For this review, take the finished solid that the model builds, in its own axes (mm). A direction names the side the tool comes from. Coordinates: 2 decimals unless noted, no trailing zeros. Order: outer loops, then holes, each group sorted by start corner. A loop starts at its lowest first (then second) coordinate and runs counter-clockwise, first axis right, second up. Notation, with made-up numbers: (35.25, 55) -> (46.25, 55) arc R11 ccw to (46.25, 66) -> close; hole circle Ø10 at (29, 6.5). An arc over 180 degrees is marked (long way). Answer as a JSON object with one key per item and string values. Group by question number.
1) Add section C-C, the plane z = -45.5. Write out the cut boundary in (x, y), then the cut area to 3 significant figures.
2) Machinability: for faces 1 (the flat face through (12, 22, -23)), 2 (the flat face through (0, 10, -62)), 3 (the flat face through (6, 20, -96)), which of the approach directions +Z, -Z, +X, -X, +Y, -Y give a long, thin tool a straight path to every point of the face, cutting with its end or side? Answer none if there is none.
3) Add section A-A, the plane y = 17. Write out the cut boundary in (x, z).
4) Draft analysis for pull direction Z (two halves, no side actions). For faces 4 (the flat face through (125, 13, -126)), 5 (the flat face through (125, 27, -5)), 6 (the flat face through (6, 20, -30)), state which applies: +Z half, -Z half, draft (parallel to the pull), parting line (faces both ways), or undercut.
5) Wall thickness on L1, parallel to X at y = 23.25, z = -28.5; L2, parallel to Z at x = 67, y = 25.5; L3, parallel to Z at x = 108.5, y = 17.5: over which ranges is each line inside the solid? List them lowest first.
6) For pin 1 (7 mm diameter, centred on x = 155, z = -17.5, fed in from +Y); pin 2 (12 mm diameter, centred on x = 116, z = -75, fed in from +Y), all flat-tipped, find the tip position at first contact; note any pin that passes through.
7) Add section B-B, the plane x = 154.5. Write out the cut boundary in (y, z).
from build123d import *

# Parameters (mm, degrees)
SKETCH1_W           = 253
SKETCH1_H           = 126
BOSS_EXTRUDE1_DEPTH = 27
SKETCH2_W           = 229
SKETCH2_H           = 102
CUT_EXTRUDE1_DEPTH  = 7
SKETCH3_W           = 229
SKETCH3_H           = 85
CUT_EXTRUDE2_DEPTH  = 7
SKETCH4_W           = 12
SKETCH4_H           = 66
CUT_EXTRUDE3_DEPTH  = 14
SKETCH5_W           = 12
SKETCH5_H           = 66
CUT_EXTRUDE4_DEPTH  = 14
CUT_EXTRUDE5_DEPTH  = 7
FILLET1_R           = 2.5


with BuildPart() as part:
    # Sketch1 → Boss-Extrude1 (new body)
    with BuildSketch(Plane(origin=(0, 0, 0), x_dir=(1, 0, 0), z_dir=(0, 1, 0))):
        with Locations((126.5, 63)):
            Rectangle(SKETCH1_W, SKETCH1_H)
    extrude(amount=BOSS_EXTRUDE1_DEPTH)

    # Sketch2 → Cut-Extrude1 (cut)
    with BuildSketch(Plane(origin=(0, 27, 0), x_dir=(1, 0, 0), z_dir=(0, 1, 0))):
        with Locations((126.5, 63)):
            Rectangle(SKETCH2_W, SKETCH2_H)
    extrude(amount=-CUT_EXTRUDE1_DEPTH, mode=Mode.SUBTRACT)

    # Sketch3 → Cut-Extrude2 (cut)
    with BuildSketch(Plane(origin=(0, 20, 0), x_dir=(1, 0, 0), z_dir=(0, 1, 0))):
        with Locations((126.5, 63)):
            Rectangle(SKETCH3_W, SKETCH3_H)
    extrude(amount=-CUT_EXTRUDE2_DEPTH, mode=Mode.SUBTRACT)

    # Sketch4 → Cut-Extrude3 (cut)
    with BuildSketch(Plane(origin=(0, 27, 0), x_dir=(1, 0, 0), z_dir=(0, 1, 0))):
        with Locations((6, 63)):
            Rectangle(SKETCH4_W, SKETCH4_H)
    extrude(amount=-CUT_EXTRUDE3_DEPTH, mode=Mode.SUBTRACT)

    # Sketch5 → Cut-Extrude4 (cut)
    with BuildSketch(Plane(origin=(0, 27, 0), x_dir=(1, 0, 0), z_dir=(0, 1, 0))):
        with Locations((247, 63)):
            Rectangle(SKETCH5_W, SKETCH5_H)
    extrude(amount=-CUT_EXTRUDE4_DEPTH, mode=Mode.SUBTRACT)

    # Sketch6 → Cut-Extrude5 (cut)
    with BuildSketch(Plane(origin=(0, 27, 0), x_dir=(1, 0, 0), z_dir=(0, 1, 0))):
        with BuildLine():
            Line((12, 12), (17, 12))
            ThreePointArc((17, 12), (14.5, 9.5), (12, 12))
        make_face()
        with BuildLine():
            Line((236, 12), (241, 12))
            ThreePointArc((241, 12), (238.5, 9.5), (236, 12))
        make_face()
        with BuildLine():
            Line((12, 114), (17, 114))
            ThreePointArc((17, 114), (14.5, 116.5), (12, 114))
        make_face()
        with BuildLine():
            Line((236, 114), (241, 114))
            ThreePointArc((241, 114), (238.5, 116.5), (236, 114))
        make_face()
    extrude(amount=-CUT_EXTRUDE5_DEPTH, mode=Mode.SUBTRACT)

    # Fillet1
    fillet1_edges = [part.edges().sort_by_distance(p)[0] for p in [
        (241, 16.5, -105.5),
        (241, 16.5, -20.5),
        (12, 16.5, -20.5),
        (12, 16.5, -105.5),
    ]]
    fillet(fillet1_edges, radius=FILLET1_R)


solid = part.part
Output values:
{
 "1": {"outline": "(0, 0) -> (253, 0) -> (253, 13) -> (0, 13) -> close", "area": "3,290 mm²"},
 "2": {"face 1": "+Y", "face 2": "+Z, -Z, -X, +Y, -Y", "face 3": "+X, -X, +Y"},
 "3": {"outline": "(0, -126) -> (253, -126) -> (253, -96) -> (241, -96) -> (241, -103) arc R2.5 cw to (238.5, -105.5) -> (14.5, -105.5) arc R2.5 cw to (12, -103) -> (12, -96) -> (0, -96) -> close; (0, -30) -> (12, -30) -> (12, -23) arc R2.5 cw to (14.5, -20.5) -> (238.5, -20.5) arc R2.5 cw to (241, -23) -> (241, -30) -> (253, -30) -> (253, 0) -> (0, 0) -> close"},
 "4": {"face 4": "-Z half", "face 5": "draft", "face 6": "undercut"},
 "5": {"L1": "x = 0 to 12, 241 to 253", "L2": "z = -126 to -114, -12 to 0", "L3": "z = -126 to -105.5, -20.5 to 0"},
 "6": {"pin 1": "stops at y = 20", "pin 2": "stops at y = 13"},
 "7": {"outline": "(0, -126) -> (27, -126) -> (27, -114) -> (20, -114) -> (20, -105.5) -> (13, -105.5) -> (13, -20.5) -> (20, -20.5) -> (20, -12) -> (27, -12) -> (27, 0) -> (0, 0) -> close"}
}
